Input: part model. Units: mm. Frame: model coordinates. Face numbers are marked on the shaded views. Coordinates: 2 decimals unless noted, no trailing zeros. Write each loop counter-clockwise with the first axis right and the second up, starting at its lowest first coordinate (ties: lowest second). Pieces come first, ordered by that corner, then holes. Notation, with made-up numbers: (-37.5, 55.5) - (7.5, 55.5) arc R25 ccw to (7.5, 90.5) - close; hole circle Ø2 at (84.5, 61). An arc over 180 degrees is marked (long way). Use a Markdown table: item, result. Add a question column.
Q1. Mould query, pull axis X, two halves, no side actions, for the marked faces 1, 2 and 3. Classes: released by +X, released by -X, zero draft, split by the parting line, or undercut.
Q2. Section query D-D (x = -5). Return the cut outline in (y, z), then the cut area to 3 significant figures.
Q3. Pin query (flat end, axial travel): P1, Ø8, axis at x = -12.5, z = -8, coming from the -Y side; P2, Ø1.5, axis at x = 8, z = -69, coming from the +Y side; P3, Ø1, axis at x = 10.5, z = -162, coming from the +Y side. Return the tip coordinate at first contact, or that it passes through.
Q4. Section query B-B (y = -30). Return the cut outline in (x, z).
Q5. Material intervals for probe 1 along Z at (x, y) = (6, -39); probe 2 along X at (y, z) = (-25, -123); probe 3 along Y at (x, z) = (0, -145.5), sorted ascending. Write a range as from..to.
Q6. Section query C-C (z = -11.5). Return the cut outline in (x, y).
Q7. Section query A-A (z = -182). Return the cut outline in (x, y).
from build123d import *

# Parameters (mm, degrees)
BOSS_EXTRUDE1_DEPTH      = 12.7
BOSS_EXTRUDE1_DEPTH_BACK = 215.9
SKETCH1_R                = 16.51
SHELL1_T                 = 1.27
SKETCH2_W                = 17.94421574
SKETCH2_H                = 13.769076435
CUT_EXTRUDE1_DEPTH       = 114.3
SKETCH3_W                = 20.21918521
SKETCH3_H                = 3.109812076
BOSS_EXTRUDE2_DEPTH      = 12.7
FILLET1_R                = 10.16


with BuildPart() as part:
    # Sketch1 → Boss-Extrude1 (new, two sides: drawn at the far end of the back side and taken through both)
    with BuildSketch(Plane.XY.offset(-BOSS_EXTRUDE1_DEPTH_BACK)):
        with Locations((0, -25.4)):
            Circle(SKETCH1_R)
    extrude(amount=BOSS_EXTRUDE1_DEPTH + BOSS_EXTRUDE1_DEPTH_BACK)

    # Shell1 (no face opened: a closed hollow body)
    add(offset(amount=-SHELL1_T, mode=Mode.PRIVATE), mode=Mode.SUBTRACT)

    # Sketch2 → Cut-Extrude1 (cut)
    with BuildSketch(Plane.XY):
        with Locations((-0.977160263, -11.097927059)):
            Rectangle(SKETCH2_W, SKETCH2_H)
    extrude(amount=-CUT_EXTRUDE1_DEPTH, mode=Mode.SUBTRACT)

    # Sketch3 → Boss-Extrude2 (add)
    with BuildSketch(Plane.XY.offset(12.7)):
        with Locations((0, -25.4)):
            Rectangle(SKETCH3_W, SKETCH3_H)
    extrude(amount=BOSS_EXTRUDE2_DEPTH)

    # Fillet1
    # the kernel refuses this fillet: 10.16 mm, written as the material it takes off along each edge
    with BuildSketch(Plane(origin=(10.109592605, -52.354906038, 25.4), x_dir=(0, 0, -1), z_dir=(0, 1, 0)), Plane(origin=(-10.109592605, 1.554906038, 25.4), x_dir=(0, 0, -1), z_dir=(0, -1, 0))) as fillet1_piece_1:
        with BuildLine():
            CenterArc((FILLET1_R, FILLET1_R), FILLET1_R, 180, 90)
            Line((0, FILLET1_R), (0, 0))
            Line((0, 0), (FILLET1_R, 0))
        make_face()
    extrude(amount=53.909812076, mode=Mode.SUBTRACT)


solid = part.part
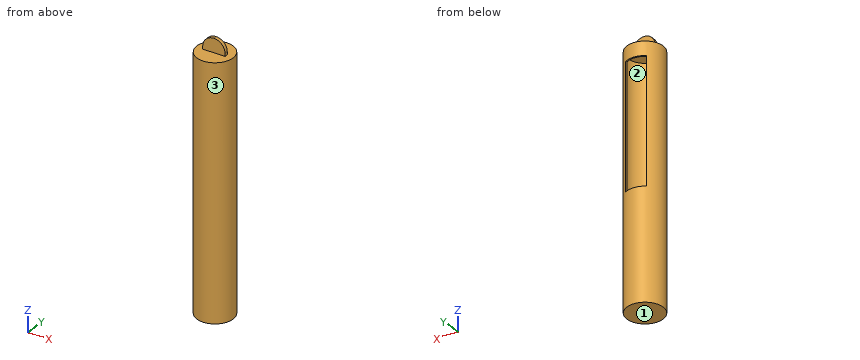
Values follow:
| question | item | result |
|---|---|---|
| 1 | face 1 | zero draft |
| 1 | face 2 | undercut |
| 1 | face 3 | split by the parting line |
| 2 | outline | (-41.13, -215.9) - (-9.67, -215.9) - (-9.67, -114.3) - (-11, -114.3) - (-11, -214.63) - (-39.8, -214.63) - (-39.8, 11.43) - (-11, 11.43) - (-11, 0) - (-9.67, 0) - (-9.67, 12.7) - (-23.85, 12.7) - (-23.85, 24.06) - (-26.95, 24.06) - (-26.95, 12.7) - (-41.13, 12.7) - close |
| 2 | area | 567 mm2 |
| 3 | P1 | y = -39.55 |
| 3 | P2 | y = -10.95 |
| 3 | P3 | y = -12.26 |
| 4 | outline | (-15.86, -215.9) - (15.86, -215.9) - (15.86, 12.7) - (-15.86, 12.7) - close; hole (-14.53, -214.63) - (14.53, -214.63) - (14.53, 11.43) - (-14.53, 11.43) - close |
| 5 | probe 1 | -215.9..-214.63, 11.43..12.7 |
| 5 | probe 2 | -16.51..-15.23, 15.23..16.51 |
| 5 | probe 3 | -41.91..-40.64, -10.16..-8.89 |
| 6 | outline | (-9.95, -13.86) - (-9.95, -12.22) arc R16.51 ccw (long way) to (7.99, -10.95) - (7.99, -12.43) arc R15.24 cw (long way) to start |
| 7 | outline | circle Ø33.02 at (0, -25.4); hole circle Ø30.48 at (0, -25.4) |
